Read the model definition and answer for the solid it produces. Units are mm, in the model's axes. Give positions to 0.01 mm unless a question says otherwise; leave off trailing zeros. Order: outer loops, then holes, each group sorted by start corner. A loop starts at its lowest first (then second) coordinate and runs counter-clockwise, first axis right, second up. Notation, with made-up numbers: (-12, 6.25) - (19, 6.25) arc R10 ccw to (19, 11.25) - close; hole circle Ø8 at (-11, 77). An arc over 180 degrees is marked (long way). Return JSON: item names as keys, results as strings.
```python
from build123d import *

# Parameters (mm, degrees)
SKETCH1_W                = 3
SKETCH1_H                = 10
BOSS_EXTRUDE2_DEPTH      = 3
F_6_0_6_DIAMETER_HOLE1_D = 6
SKETCH5_W                = 105
SKETCH5_H                = 117
CUT_EXTRUDE1_DEPTH       = 10


with BuildPart() as part:
    # Sketch1 → Boss-Extrude2 (new body)
    with BuildSketch(Plane.XY):
        Polygon((-5, 65), (5, 65), (5, 62), (45, 62), (45, 65), (55, 65), (55, 62), (75, 62), (75, 12.5), (81.5, 12.5), (81.5, -12.5), (75, -12.5), (75, -100), (65, -100), (65, -103), (55, -103), (55, -100), (35, -100), (35, -103), (25, -103), (25, -100), (5, -100), (5, -103), (-5, -103), (-5, -100), (-25, -100), (-25, -103), (-35, -103), (-35, -100), (-55, -100), (-55, -103), (-65, -103), (-65, -100), (-75, -100), (-75, -12.5), (-81.5, -12.5), (-81.5, 12.5), (-75, 12.5), (-75, 62), (-55, 62), (-55, 65), (-45, 65), (-45, 62), (-5, 62), align=None)
        with Locations((-73.5, 0)):
            Rectangle(SKETCH1_W, SKETCH1_H, mode=Mode.SUBTRACT)
        with Locations((73.5, 0)):
            Rectangle(SKETCH1_W, SKETCH1_H, mode=Mode.SUBTRACT)
    extrude(amount=BOSS_EXTRUDE2_DEPTH)

    # Ø6.0 (6) Diameter Hole1 (through all)
    with Locations(Plane.XY.offset(3)):
        with Locations((-60, 47), (60, 47), (-60, -85), (60, -85)):
            Hole(F_6_0_6_DIAMETER_HOLE1_D / 2)

    # Sketch5 → Cut-Extrude1 (cut)
    with BuildSketch(Plane.XY.offset(3)):
        with Locations((0, -19)):
            Rectangle(SKETCH5_W, SKETCH5_H)
    extrude(amount=-CUT_EXTRUDE1_DEPTH, mode=Mode.SUBTRACT)


solid = part.part
```
Q1. Determine the mould class of faces 1 (the cylindrical face through (-57.6, -86.8, 1.5)), 2 (the flat face through (-53, -18, 3)) for opening direction X: released by +X, released by -X, zero draft, split by the parting line, or undercut.
Values:
{"face 1": "undercut", "face 2": "zero draft"}
Q2. A cutting plane is placed at B-B (y = 47). Write down the section's boundary in (x, z), and give its area (3 significant figures).
Values:
{"outline": "(-75, 0) - (-63, 0) - (-63, 3) - (-75, 3) - close; (-57, 0) - (57, 0) - (57, 3) - (-57, 3) - close; (63, 0) - (75, 0) - (75, 3) - (63, 3) - close", "area": "414 mm²"}
Q3. A cutting plane is placed at D-D (y = -26). Write down the section's boundary in (x, z), and give its area (3 significant figures).
Values:
{"outline": "(-75, 0) - (-52.5, 0) - (-52.5, 3) - (-75, 3) - close; (52.5, 0) - (75, 0) - (75, 3) - (52.5, 3) - close", "area": "135 mm²"}
Q4. Consider L1, parallel to Y at x = 60, z = 1.1; L2, parallel to X at y = -4, z = 0.95; L3, parallel to X at y = -6, z = 2.4. Determine where each line is inside the solid, lowest interval first.
Values:
{"L1": "y = -103 to -88, -82 to 44, 50 to 62", "L2": "x = -81.5 to -75, -72 to -52.5, 52.5 to 72, 75 to 81.5", "L3": "x = -81.5 to -52.5, 52.5 to 81.5"}
Q5. Given pin 1 (1.5 mm diameter, centred on y = -101, z = 1, fed in from -X); pin 2 (1.5 mm diameter, centred on x = -36, z = 2, fed in from +Y); pin 3 (5 mm diameter, centred on x = -60, y = 47, fed in from +Z); pin 4 (0.9 mm diameter, centred on x = -43.5, z = 1, fed in from -Y), each flat-ended and moving along its own axis, determine where each tip first touches the part or whether it passes through.
Values:
{"pin 1": "stops at x = -65", "pin 2": "stops at y = 62", "pin 3": "passes through", "pin 4": "stops at y = -100"}
Q6. A cutting plane is placed at C-C (x = 11.5). Write down the section's boundary in (y, z), and give its area (3 significant figures).
Values:
{"outline": "(-100, 0) - (-77.5, 0) - (-77.5, 3) - (-100, 3) - close; (39.5, 0) - (62, 0) - (62, 3) - (39.5, 3) - close", "area": "135 mm²"}
Q7. A cutting plane is placed at A-A (x = -60). Write down the section's boundary in (y, z).
Values:
{"outline": "(-103, 0) - (-88, 0) - (-88, 3) - (-103, 3) - close; (-82, 0) - (44, 0) - (44, 3) - (-82, 3) - close; (50, 0) - (62, 0) - (62, 3) - (50, 3) - close"}
